Check sheet for the modelled part. Datum: model origin and axes. Units: mm. Round coordinates to 2 decimals unless told otherwise and drop trailing zeros.
Item 1: Depth check by flat-ended pin: pin 1 (1.6 mm diameter, centred on x = 34, z = -40, fed in from -Y); pin 2 (3 mm diameter, centred on x = 11.5, z = -68.5, fed in from -Y). Enter the tip coordinate at first touch or a pass-through.
Item 2: Material ranges on line 1 along X through (y, z) = (0.5, -40); line 2 along X through (y, z) = (0.35, -40); line 3 along Z through (x, y) = (41, 0.3), recorded low to high.
Item 3: Section check B-B, the plane z = -40. State how many separate pieces and enclosed holes the cut face has, plus the area to 3 significant figures.
Item 4: Release check for a two-part mould opening along X. For faces 1 (the cylindrical face through (43.47, 0.49, -39.54)), 2 (the flat face through (48, 0, -41)), 3 (the cylindrical face through (78.57, 0.51, -78.5)) record: pulls with the +X half, pulls with the -X half, needs draft (parallel to the pull), parting line crosses it, or undercut.
from build123d import *

# Parameters (mm, degrees)
ESQUISSE1_W                  = 80
ESQUISSE1_H                  = 80
EXTRUSION1_DEPTH             = 1
CONG_1_R                     = 5
ESQUISSE2_R                  = 3.5
ENL_V_MAT_EXTRU_1_DEPTH      = 114.141504321
ESQUISSE3_R                  = 1
ENL_V_MAT_EXTRU_2_DEPTH      = 114.141504321
R_P_TITION_CIRCULAIRE1_COUNT = 2
CHANFREIN1_SIZE              = 1


with BuildPart() as part:
    # Esquisse1 → Extrusion1 (new body)
    with BuildSketch(Plane(origin=(0, 0, 0), x_dir=(1, 0, 0), z_dir=(0, 1, 0))):
        with Locations((40, 40)):
            Rectangle(ESQUISSE1_W, ESQUISSE1_H)
    extrude(amount=EXTRUSION1_DEPTH)

    # Congé1
    cong_1_edges = [part.edges().sort_by_distance(p)[0] for p in [
        (0, 0.5, -80),
        (80, 0.5, -80),
        (80, 0.5, 0),
        (0, 0.5, 0),
    ]]
    fillet(cong_1_edges, radius=CONG_1_R)

    # Esquisse2 → Enlèv. mat.-Extru.1 (cut, through all)
    with BuildSketch(Plane.XZ):
        with Locations(Location((40, -40, 0), (0, 0, 270))):
            Circle(ESQUISSE2_R)
    extrude(amount=-ENL_V_MAT_EXTRU_1_DEPTH, mode=Mode.SUBTRACT)

    # Esquisse3 → Enlèv. mat.-Extru.2 (cut, through all)
    with BuildSketch(Plane(origin=(0, 1, 0), x_dir=(1, 0, 0), z_dir=(0, 1, 0))):
        with Locations(Location((34, 40, 0), (0, 0, 270))):
            Circle(ESQUISSE3_R)
    enl_v_mat_extru_2 = extrude(amount=-ENL_V_MAT_EXTRU_2_DEPTH, mode=Mode.SUBTRACT)

    # Répétition circulaire1: Enlèv. mat.-Extru.2 ×2 about axis
    r_p_tition_circulaire1_axis = Axis((40, 0, -40), (0, 1, 0))
    for i in range(1, R_P_TITION_CIRCULAIRE1_COUNT):
        add(enl_v_mat_extru_2.rotate(r_p_tition_circulaire1_axis, i * 360 / R_P_TITION_CIRCULAIRE1_COUNT), mode=Mode.SUBTRACT)

    # Chanfrein1
    chanfrein1_edges = [part.edges().sort_by_distance(p)[0] for p in [
        (34, 0, -41),
        (46, 0, -39),
    ]]
    chamfer(chanfrein1_edges, length=CHANFREIN1_SIZE - 0.0001)  # a hair under: the kernel refuses the full size


solid = part.part
Values found:
1. pin 1: passes through
1. pin 2: stops at y = 0
2. line 1: x = 0 to 32.5, 35.5 to 36.5, 43.5 to 44.5, 47.5 to 80
2. line 2: x = 0 to 32.35, 35.65 to 36.5, 43.5 to 44.35, 47.65 to 80
2. line 3: z = -80 to -43.35, -36.65 to 0
3. separate pieces: 4
3. enclosed holes: 0
3. area: 67.0 mm2
4. face 1: undercut
4. face 2: needs draft
4. face 3: pulls with the +X half
